Check sheet for the modelled part. Datum: model origin and axes. Units: mm. Round coordinates to 2 decimals unless told otherwise and drop trailing zeros. Order: outer loops, then holes, each group sorted by start corner. A loop starts at its lowest first (then second) coordinate and runs counter-clockwise, first axis right, second up. Notation, with made-up numbers: (-19, 12) -> (2, 12) arc R18 ccw to (2, 43) -> close; hole circle Ø8 at (49, 56). An arc over 180 degrees is marked (long way). Answer in a Markdown table with one row per item. Add a question column.
1. Sectioned sample at A-A, the plane x = 44.45. Record the boundary of the cut face in (y, z).
2. Sectioned sample at B-B, the plane z = -72.5. Record the boundary of the cut face in (x, y), then the cut area to 3 significant figures.
3. Material ranges on L1, parallel to Z at x = 44.45, y = 3; L2, parallel to Z at x = 81.5, y = 7.5 (3 decimals); L3, parallel to Z at x = 6.5, y = 9, recorded low to high. Write a range as from..to.
4. Depth check by flat-ended pin: P1, Ø5, axis at x = 37.5, y = 9.5, coming from the -Z side; P2, Ø8, axis at x = 44.45, z = -15.875, coming from the +Y side; P3, Ø11, axis at x = 44.45, z = -111.125, coming from the +Y side. Enter the tip coordinate at first touch or a pass-through.
```python
from build123d import *

# Parameters (mm, degrees)
SKETCH1_W                                        = 88.9
SKETCH1_H                                        = 127
BOSS_EXTRUDE1_DEPTH                              = 12.7
CSK_FOR_1_4_FLAT_HEAD_MACHINE_SCREW1_D           = 6.7564
CSK_FOR_1_4_FLAT_HEAD_MACHINE_SCREW1_CSINK_D     = 15.5273756
CSK_FOR_1_4_FLAT_HEAD_MACHINE_SCREW1_CSINK_ANGLE = 82
FILLET1_R                                        = 6.35
FILLET2_R                                        = 6.35


with BuildPart() as part:
    # Sketch1 → Boss-Extrude1 (new body)
    with BuildSketch(Plane(origin=(0, 0, 0), x_dir=(1, 0, 0), z_dir=(0, 1, 0))):
        with Locations((44.45, 63.5)):
            Rectangle(SKETCH1_W, SKETCH1_H)
    extrude(amount=BOSS_EXTRUDE1_DEPTH)

    # CSK for 1/4 Flat Head Machine Screw1 (through all)
    with Locations(Plane(origin=(0, 12.7, 0), x_dir=(-1, 0, 0), z_dir=(0, 1, 0))):
        with Locations((-44.45, -15.875), (-44.45, -111.125)):
            CounterSinkHole(CSK_FOR_1_4_FLAT_HEAD_MACHINE_SCREW1_D / 2, CSK_FOR_1_4_FLAT_HEAD_MACHINE_SCREW1_CSINK_D / 2, counter_sink_angle=CSK_FOR_1_4_FLAT_HEAD_MACHINE_SCREW1_CSINK_ANGLE)

    # Fillet1
    fillet1_edges = [part.edges().sort_by_distance(p)[0] for p in [
        (0, 6.35, -127),
        (88.9, 6.35, -127),
        (88.9, 6.35, 0),
        (0, 6.35, 0),
    ]]
    fillet(fillet1_edges, radius=FILLET1_R)

    # Fillet2
    fillet2_edges = [part.edges().sort_by_distance(p)[0] for p in [
        (44.45, 12.7, 0),
        (0, 12.7, -63.5),
        (88.9, 12.7, -63.5),
        (44.45, 12.7, -127),
        (87.040128061, 12.7, -125.140128061),
        (87.040128061, 12.7, -1.859871939),
        (1.859871939, 12.7, -125.140128061),
        (1.859871939, 12.7, -1.859871939),
    ]]
    fillet(fillet2_edges, radius=FILLET2_R)


solid = part.part
```
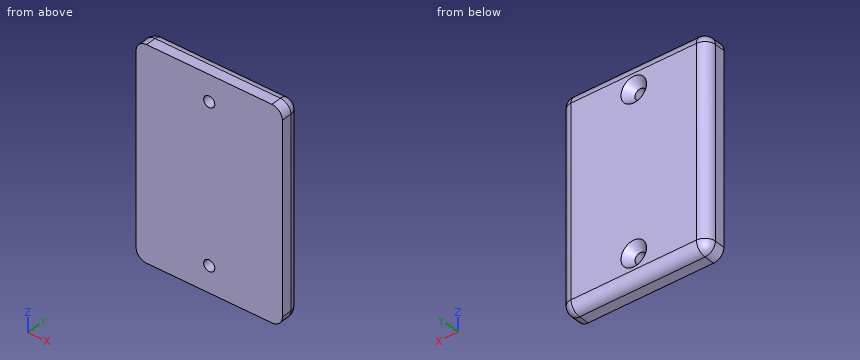
Answer key:
| question | item | result |
|---|---|---|
| 1 | outline | (0, -127) -> (6.35, -127) arc R6.35 ccw to (12.7, -120.65) -> (12.7, -118.89) -> (7.66, -114.5) -> (0, -114.5) -> close; (0, -107.75) -> (7.66, -107.75) -> (12.7, -103.36) -> (12.7, -23.64) -> (7.66, -19.25) -> (0, -19.25) -> close; (0, -12.5) -> (7.66, -12.5) -> (12.7, -8.11) -> (12.7, -6.35) arc R6.35 ccw to (6.35, 0) -> (0, 0) -> close |
| 2 | outline | (0, 0) -> (88.9, 0) -> (88.9, 6.35) arc R6.35 ccw to (82.55, 12.7) -> (6.35, 12.7) arc R6.35 ccw to (0, 6.35) -> close |
| 2 | area | 1,110 mm² |
| 3 | L1 | z = -127..-114.5, -107.75..-19.25, -12.5..0 |
| 3 | L2 | z = -126.895..-0.105 |
| 3 | L3 | z = -126.42..-0.58 |
| 4 | P1 | stops at z = -126.97 |
| 4 | P2 | stops at y = 8.37 |
| 4 | P3 | stops at y = 10.1 |
